Model file for the job. Use its own axes, mm. Face numbers are marked on the shaded views. A direction names the side the tool comes from. Round coordinates to 2 decimals unless told otherwise and drop trailing zeros. Loops run counter-clockwise (first coordinate to the right, second up) from the corner with the lowest first, then second, coordinate; pieces in that order, holes last. Notation, with made-up numbers: (60, -25.5) - (118, -25.5) arc R25 cw to (118, 8.5) - close; hole circle Ø2 at (-32.5, 50). An arc over 180 degrees is marked (long way). Use one line per item in the form item = value.
from build123d import *

# Parameters (mm, degrees)
BOSS_EXTRUDE1_DEPTH = 50.8
FILLET1_R           = 3.175


with BuildPart() as part:
    # Sketch1 → Boss-Extrude1 (new body)
    with BuildSketch(Plane(origin=(0, 0, 0), x_dir=(1, 0, 0), z_dir=(0, 1, 0))):
        Polygon((-64.29375, 47.625), (-63.5, 47.625), (-63.5, 0), (63.5, 0), (63.5, 47.625), (64.29375, 47.625), (64.29375, -0.79375), (-64.29375, -0.79375), align=None)
    extrude(amount=BOSS_EXTRUDE1_DEPTH)

    # Fillet1
    fillet1_edges = [part.edges().sort_by_distance(p)[0] for p in [
        (-63.5, 25.4, 0),
        (63.5, 25.4, 0),
        (64.29375, 25.4, 0.79375),
        (-64.29375, 25.4, 0.79375),
    ]]
    fillet(fillet1_edges, radius=FILLET1_R)


solid = part.part
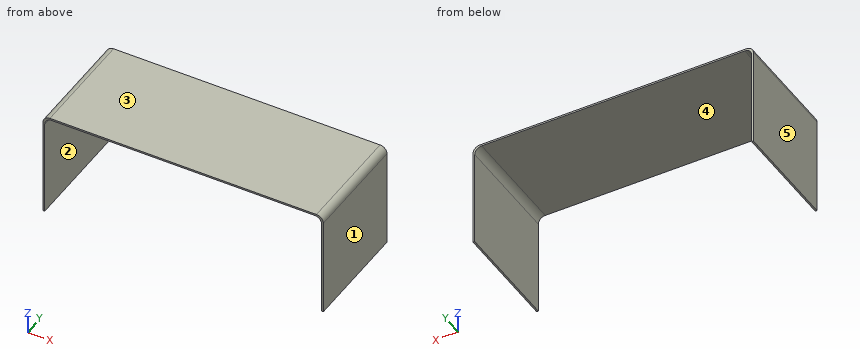
1. Cut at A-A, the plane z = -7. Give the cut face in (x, y).
Geometry check:
outline = (-64.29, 0) - (-63.5, 0) - (-63.5, 50.8) - (-64.29, 50.8) - close; (63.5, 0) - (64.29, 0) - (64.29, 50.8) - (63.5, 50.8) - close
2. Flat gauge pin, fed straight in: pin 1 (1.5 mm diameter, centred on x = 49, y = 26, fed in from -Z). Where does the tip first touch, or does it go through?
Geometry check:
pin_1 = 0
3. Wall check: probe 1 along X at (y, z) = (25, -42.5); probe 2 along Z at (x, y) = (-18, 8). Give the ranges that are in metal, low to high.
Geometry check:
probe_1 = -64.29 to -63.5, 63.5 to 64.29
probe_2 = 0 to 0.79
4. Pull direction X, two halves, no side cores. Call the marked faces 3, 4 and 5: +X half, -X half, draft (parallel to the pull), parting line (faces both ways), or undercut.
Geometry check:
face_3 = draft
face_4 = undercut
face_5 = -X half
5. Cut at B-B, the plane y = 11. Give the cut face in (x, z) (3 decimals).
Geometry check:
outline = (-64.294, -47.625) - (-63.5, -47.625) - (-63.5, -3.175) arc R3.175 cw to (-60.325, 0) - (60.325, 0) arc R3.175 cw to (63.5, -3.175) - (63.5, -47.625) - (64.294, -47.625) - (64.294, -2.381) arc R3.175 ccw to (61.119, 0.794) - (-61.119, 0.794) arc R3.175 ccw to (-64.294, -2.381) - close
6. Tool access for the marked faces 1 and 2: list every direction of +Z, -Z, +X, -X, +Y, -Y with a clear straight run to the whole face (end or side of a thin tool).
Geometry check:
face_1 = +Z, -Z, +X, +Y, -Y
face_2 = -Z, +Y, -Y
7. Cut at C-C, the plane x = 31. Give the cut face in (y, z).
Geometry check:
outline = (0, 0) - (50.8, 0) - (50.8, 0.79) - (0, 0.79) - close
